```python
from build123d import *

# Parameters (mm, degrees)
SKETCH1_R           = 34.0741
SKETCH1_R_2         = 30.1625
BOSS_EXTRUDE1_DEPTH = 63.5
BOSS_EXTRUDE2_START = -30.95625
SKETCH2_R           = 30.1625
SKETCH2_R_2         = 26.035
BOSS_EXTRUDE2_DEPTH = 1.5875


with BuildPart() as part:
    # Sketch1 → Boss-Extrude1 (new body)
    with BuildSketch(Plane(origin=(0, 0, 0), x_dir=(0, 0, -1), z_dir=(1, 0, 0))):
        Circle(SKETCH1_R)
        Circle(SKETCH1_R_2, mode=Mode.SUBTRACT)
    extrude(amount=BOSS_EXTRUDE1_DEPTH)

    # Sketch2 → Boss-Extrude2 (add)
    with BuildSketch(Plane(origin=(63.5, 0, 0), x_dir=(0, 0, -1), z_dir=(1, 0, 0)).offset(BOSS_EXTRUDE2_START)):
        Circle(SKETCH2_R)
        Circle(SKETCH2_R_2, mode=Mode.SUBTRACT)
    extrude(amount=BOSS_EXTRUDE2_DEPTH)


solid = part.part
```
Work out the finished part from the listing and answer in its coordinate system (mm). A direction names the side the tool comes from. Coordinates: 2 decimals unless noted, no trailing zeros. Order: outer loops, then holes, each group sorted by start corner. A loop starts at its lowest first (then second) coordinate and runs counter-clockwise, first axis right, second up. Notation, with made-up numbers: (70.25, 15.25) - (100.25, 15.25) arc R14 ccw to (100.25, 35.25) - close; hole circle Ø5 at (27.5, 65). An arc over 180 degrees is marked (long way). Answer as a JSON object with one key per item and string values.
1. Find section D-D on y = 27. Determine the outline of the cut face in (x, z).
Output values:
{"outline": "(0, -20.79) - (63.5, -20.79) - (63.5, -13.45) - (34.13, -13.45) - (34.13, 13.45) - (63.5, 13.45) - (63.5, 20.79) - (0, 20.79) - (0, 13.45) - (32.54, 13.45) - (32.54, -13.45) - (0, -13.45) - close"}
2. Find section C-C on x = 21.5. Determine the outline of the cut face in (y, z) (1 decimal).
Output values:
{"outline": "circle Ø68.1 at (0, 0); hole circle Ø60.3 at (0, 0)"}
3. Find section A-A on z = 0. Determine the outline of the cut face in (x, y) (1 decimal).
Output values:
{"outline": "(0, -34.1) - (63.5, -34.1) - (63.5, -30.2) - (34.1, -30.2) - (34.1, -26) - (32.5, -26) - (32.5, -30.2) - (0, -30.2) - close; (0, 30.2) - (32.5, 30.2) - (32.5, 26) - (34.1, 26) - (34.1, 30.2) - (63.5, 30.2) - (63.5, 34.1) - (0, 34.1) - close"}
4. The mould has two halves that part along Z. Classify faces 1 (the face through (31.306, -33.264, 7.387)), 2 (the face through (16.044, 1.326, 30.133)), 3 (the face through (63.5, -28, -12)): +Z half, -Z half, draft (parallel to the pull), parting line (faces both ways), or undercut.
Output values:
{"face 1": "parting line", "face 2": "undercut", "face 3": "draft"}
5. Consider line 1 (Y direction, x = 45.75, z = 0); line 2 (Z direction, x = 21, y = -1); line 3 (Y direction, x = 33, z = 0) (3 decimals). Determine where each line is inside the solid, lowest interval first.
Output values:
{"line 1": "y = -34.07 to -30.16, 30.16 to 34.07", "line 2": "z = -34.06 to -30.15, 30.15 to 34.06", "line 3": "y = -34.074 to -26.035, 26.035 to 34.074"}
6. A tool of negligible diameter and unlimited length cuts with its end or side. For faces 4 (the face through (0, -28, -12)), 5 (the face through (34.131, -9, 25)), 6 (the face through (32.544, -9, 25)), from which of +Z, -Z, +X, -X, +Y, -Y can it reach the whole face along a straight path? Write none if from no direction.
Output values:
{"face 4": "+Z, -Z, -X, +Y, -Y", "face 5": "+X", "face 6": "-X"}
7. Each of these flat-tipped pins is pushed along its axis until it touches: P1, Ø1, axis at x = 16.5, z = 26, coming from the +Y side; P2, Ø8, axis at x = 43.5, z = -9, coming from the +Y side; P3, Ø1, axis at x = 52, z = 22, coming from the +Y side. Where does it stop, or does it pass through?
Output values:
{"P1": "stops at y = 22.6", "P2": "stops at y = 33.71", "P3": "stops at y = 26.43"}
